Drawing for the job (mm, zero at the part's lowest x, y, z). Give positions to 0.01 mm unless a question says otherwise; leave off trailing zeros. Loops run counter-clockwise (first coordinate to the right, second up) from the corner with the lowest first, then second, coordinate; pieces in that order, holes last. Notation, with made-up numbers: (-12.75, 74.25) - (13.25, 74.25) arc R28 cw to (13.25, 93.25) - close; hole circle Ø9 at (50, 5). An arc over 180 degrees is marked (long way). Return JSON: item names as keys, results as strings. Group by question number.
1) Slice it at C-C (z = 13.75). List the corners of the cut face in (x, y), and give its area (3 significant figures).
2) Slice it at B-B (y = 0.5). List the corners of the cut face in (x, z), and give its area (3 significant figures).
3) Mould opens along Z. For the marked faces 1, 2 and 3 say: released by +Z, released by -Z, zero draft, split by the parting line, or undercut.
4) Slice it at A-A (x = 10). List the corners of the cut face in (y, z).
5) Drill centre lines: probe 1 along Z at (x, y) = (10, 7); probe 2 along Z at (x, y) = (6.25, 6.75); probe 3 along X at (y, z) = (1.5, 12). Where is each one in solid material? Low to high. Write a range as from..to.
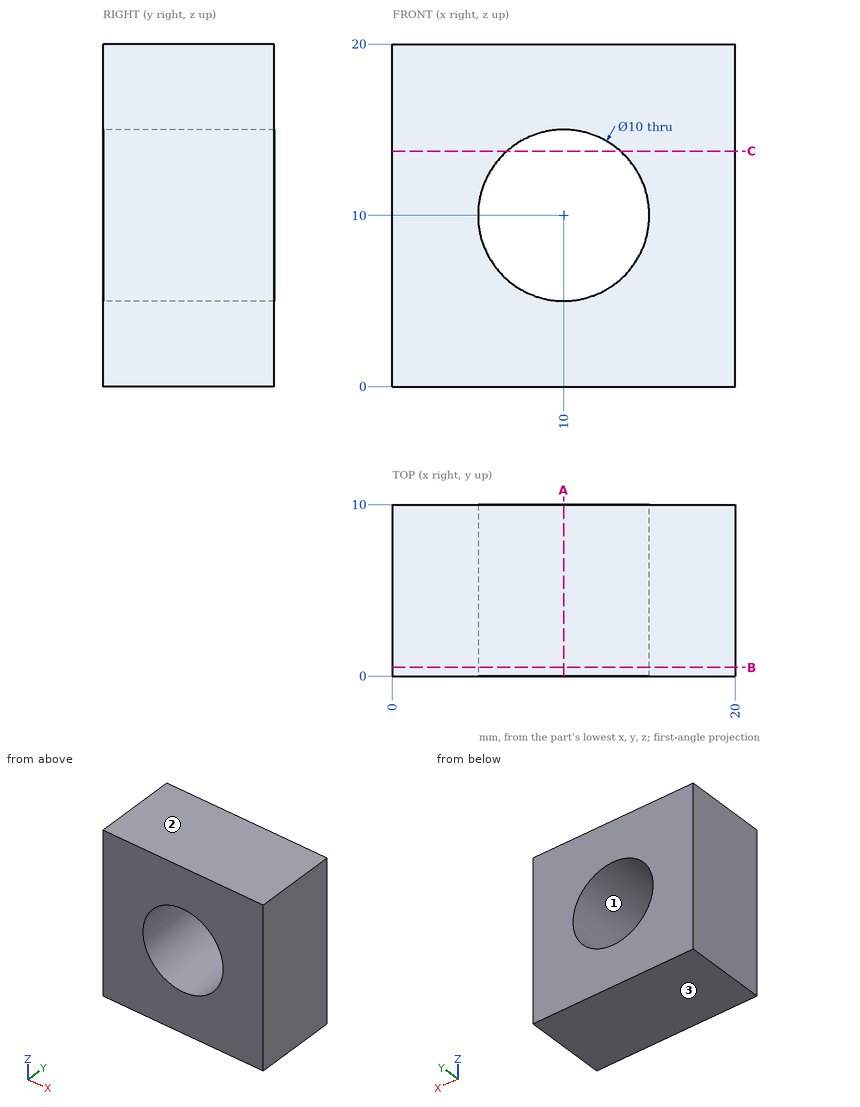
Results:
{
 "1": {"outline": "(0, 0) - (6.69, 0) - (6.69, 10) - (0, 10) - close; (13.31, 0) - (20, 0) - (20, 10) - (13.31, 10) - close", "area": "134 mm2"},
 "2": {"outline": "(0, 0) - (20, 0) - (20, 20) - (0, 20) - close; hole circle Ø10 at (10, 10)", "area": "321 mm2"},
 "3": {"face 1": "undercut", "face 2": "released by +Z", "face 3": "released by -Z"},
 "4": {"outline": "(0, 0) - (10, 0) - (10, 5) - (0, 5) - close; (0, 15) - (10, 15) - (10, 20) - (0, 20) - close"},
 "5": {"probe 1": "0..5, 15..20", "probe 2": "0..6.69, 13.31..20", "probe 3": "0..5.42, 14.58..20"}
}
